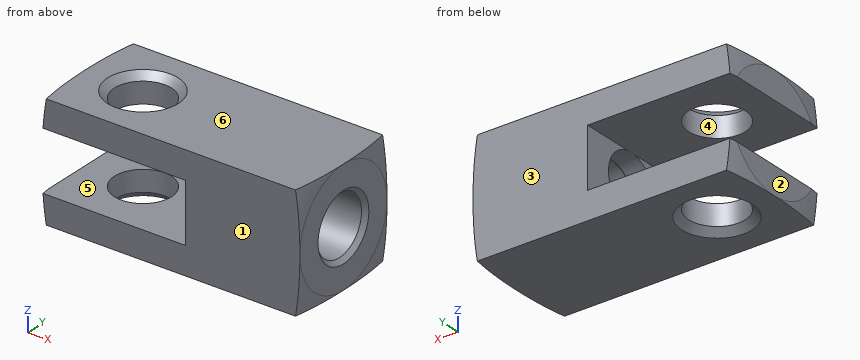
Autodesk Inventor part; units mm, degrees
ref_plane "dummy_XY" through (0, 0, 0) normal (0, 0, 1) x (1, 0, 0)
ref_plane "dummy_YZ" through (0, 0, 0) normal (1, 0, 0) x (0, 1, 0)
ref_plane "dummy_ZX" through (0, 0, 0) normal (0, 1, 0) x (0, 0, 1)
sketch "Sketch_1" plane through (0, 0, 0) normal (0, 0, 1) x (1, 0, 0)
  line L0 (-9.5504, 9.525) -> (-9.5504, -9.525)
  line L1 (-9.5504, -9.525) -> (33.3248, -9.525)
  line L2 (33.3248, -9.525) -> (33.3248, 9.525)
  line L3 (33.3248, 9.525) -> (-9.5504, 9.525)
extrude "Extrusion1" add sketch "Sketch_1" along normal mid plane 19.05
sketch "Sketch_2" plane through (0, 0, 0) normal (0, 1, 0) x (-1, 0, 0)
  line L0 (9.5504, -4.9213) -> (9.5504, 4.9213)
  line L1 (9.5504, 4.9213) -> (-14.2748, 4.9213)
  line L2 (-14.2748, 4.9213) -> (-14.2748, -4.9213)
  line L3 (-14.2748, -4.9213) -> (9.5504, -4.9213)
extrude "Extrusion2" cut sketch "Sketch_2" along normal mid plane 19.05
sketch "Sketch3" plane through (33.3248, -9.525, 9.525) normal (1, 0, 0) x (0, 0, -1)
  point P0 (9.525, 9.525)
hole "Hole1" at (33.3248, 0, 0) direction (-1, 0, 0) diameter 9.7282 depth 15.748 countersink diameter 11.1125 countersink angle 90
sketch "Sketch4" plane through (17.5768, 0, 0) normal (1, 0, 0) x (0, 0, -1)
  point P0 (0, 0)
hole "Hole2" at (17.5768, 0, 0) direction (-1, 0, 0) diameter 9.9212 depth 3.302
sketch "Sketch_5" plane through (0, 0, 0) normal (1, 0, 0) x (0, 1, 0)
  line L0 (0, -9.525) -> (0, 9.525)
  line L1 (0, 9.525) -> (5.8674, 9.525)
  line L2 (5.8674, 9.525) -> (4.7244, 8.382)
  line L3 (4.7244, 8.382) -> (4.7244, -8.382)
  line L4 (4.7244, -8.382) -> (5.8674, -9.525)
  line L5 (5.8674, -9.525) -> (0, -9.525)
  line L6 (0, -9.525) -> (0, 9.525)
revolve "Revolution1" cut sketch "Sketch_5" angle 360 about axis through (0, 0, -9.525) along (0, 0, -1)
sketch "Sketch_9" plane through (0, 0, 0) normal (0, 0, 1) x (1, 0, 0)
  line L0 (42.8498, 0) -> (33.3248, 0)
  line L1 (33.3248, 0) -> (33.3248, 9.525)
  arc A0 (33.3248, 9.525) -> (30.7848, 19.05) centre (-3.664, 4.7625) ccw
  line L2 (30.7848, 19.05) -> (42.8498, 19.05)
  line L3 (42.8498, 19.05) -> (42.8498, 0)
  line L4 (42.8498, 0) -> (33.3248, 0)
revolve "Revolution2" cut sketch "Sketch_9" angle 360 about axis through (42.8498, 0, 0) along (1, 0, 0)
sketch "Sketch_10" plane through (0, 0, 0) normal (0, 0, 1) x (1, 0, 0)
  line L0 (-9.5504, 0) -> (-19.0754, 0)
  line L1 (-19.0754, 0) -> (-19.0754, 19.05)
  line L2 (-19.0754, 19.05) -> (-7.0104, 19.05)
  arc A0 (-7.0104, 19.05) -> (-9.5504, 9.525) centre (27.4384, 4.7625) ccw
  line L3 (-9.5504, 9.525) -> (-9.5504, 0)
  line L4 (-9.5504, 0) -> (-19.0754, 0)
revolve "Revolution3" cut sketch "Sketch_10" angle 360 about axis through (-9.5504, 0, 0) along (1, 0, 0)
ref_plane "dummy_XY" through (0, 0, 0) normal (0, 0, 1) x (1, 0, 0)
ref_plane "dummy_YZ" through (0, 0, 0) normal (1, 0, 0) x (0, 1, 0)
ref_plane "dummy_ZX" through (0, 0, 0) normal (0, 1, 0) x (0, 0, 1)
ref_plane "h1_XY" through (-9.5504, 9.525, 0) normal (0, 0, 1) x (1, 0, 0)
ref_plane "h1_YZ" through (-9.5504, 9.525, 0) normal (1, 0, 0) x (0, 1, 0)
ref_plane "h1_ZX" through (-9.5504, 9.525, 0) normal (0, 1, 0) x (0, 0, 1)
ref_plane "h2_XY" through (-9.5504, -9.525, 0) normal (0, 0, 1) x (1, 0, 0)
ref_plane "h2_YZ" through (-9.5504, -9.525, 0) normal (1, 0, 0) x (0, 1, 0)
ref_plane "h2_ZX" through (-9.5504, -9.525, 0) normal (0, 1, 0) x (0, 0, 1)
ref_plane "l1_XY" through (33.3248, 9.525, 0) normal (0, 0, 1) x (1, 0, 0)
ref_plane "l1_YZ" through (33.3248, 9.525, 0) normal (1, 0, 0) x (0, 1, 0)
ref_plane "l1_ZX" through (33.3248, 9.525, 0) normal (0, 1, 0) x (0, 0, 1)
ref_plane "l11_XY" through (33.3248, 9.525, 0) normal (0, 0, 1) x (1, 0, 0)
ref_plane "l11_YZ" through (33.3248, 9.525, 0) normal (1, 0, 0) x (0, 1, 0)
ref_plane "l11_ZX" through (33.3248, 9.525, 0) normal (0, 1, 0) x (0, 0, 1)
ref_plane "l12_XY" through (0, 9.525, 0) normal (0, 0, 1) x (1, 0, 0)
ref_plane "l12_YZ" through (0, 9.525, 0) normal (1, 0, 0) x (0, 1, 0)
ref_plane "l12_ZX" through (0, 9.525, 0) normal (0, 1, 0) x (0, 0, 1)
ref_plane "l2_XY" through (-9.5504, 9.525, 0) normal (0, 0, 1) x (1, 0, 0)
ref_plane "l2_YZ" through (-9.5504, 9.525, 0) normal (1, 0, 0) x (0, 1, 0)
ref_plane "l2_ZX" through (-9.5504, 9.525, 0) normal (0, 1, 0) x (0, 0, 1)
ref_plane "l21_XY" through (33.3248, 0, 0) normal (0, 1, 0) x (1, 0, 0)
ref_plane "l21_YZ" through (33.3248, 0, 0) normal (1, 0, 0) x (0, 0, -1)
ref_plane "l21_ZX" through (33.3248, 0, 0) normal (0, 0, -1) x (0, 1, 0)
ref_plane "l22_XY" through (14.2748, 0, 0) normal (0, 1, 0) x (1, 0, 0)
ref_plane "l22_YZ" through (14.2748, 0, 0) normal (1, 0, 0) x (0, 0, -1)
ref_plane "l22_ZX" through (14.2748, 0, 0) normal (0, 0, -1) x (0, 1, 0)
ref_plane "piston_rod_clevis_XY" through (33.3248, 0, 0) normal (1, 0, 0) x (0, 0, -1)
ref_plane "piston_rod_clevis_YZ" through (33.3248, 0, 0) normal (0, 0, -1) x (0, 1, 0)
ref_plane "piston_rod_clevis_ZX" through (33.3248, 0, 0) normal (0, 1, 0) x (1, 0, 0)
ref_plane "rod_clevis_body_XY" through (0, 0, 0) normal (0, 0, 1) x (1, 0, 0)
ref_plane "rod_clevis_body_YZ" through (0, 0, 0) normal (1, 0, 0) x (0, 1, 0)
ref_plane "rod_clevis_body_ZX" through (0, 0, 0) normal (0, 1, 0) x (0, 0, 1)
ref_plane "th1_XY" through (33.3248, 5.5563, 0) normal (0, 0, 1) x (1, 0, 0)
ref_plane "th1_YZ" through (33.3248, 5.5563, 0) normal (1, 0, 0) x (0, 1, 0)
ref_plane "th1_ZX" through (33.3248, 5.5563, 0) normal (0, 1, 0) x (0, 0, 1)
ref_plane "th2_XY" through (33.3248, -5.5563, 0) normal (0, 0, 1) x (1, 0, 0)
ref_plane "th2_YZ" through (33.3248, -5.5563, 0) normal (1, 0, 0) x (0, 1, 0)
ref_plane "th2_ZX" through (33.3248, -5.5563, 0) normal (0, 1, 0) x (0, 0, 1)
ref_plane "to_cylinder_XY" through (14.2748, 0, 0) normal (1, 0, 0) x (0, 0, -1)
ref_plane "to_cylinder_YZ" through (14.2748, 0, 0) normal (0, 0, -1) x (0, 1, 0)
ref_plane "to_cylinder_ZX" through (14.2748, 0, 0) normal (0, 1, 0) x (1, 0, 0)
ref_plane "w1_XY" through (33.3248, 0, -9.525) normal (0, 1, 0) x (1, 0, 0)
ref_plane "w1_YZ" through (33.3248, 0, -9.525) normal (1, 0, 0) x (0, 0, -1)
ref_plane "w1_ZX" through (33.3248, 0, -9.525) normal (0, 0, -1) x (0, 1, 0)
ref_plane "w11_XY" through (-9.5504, 0, -4.9213) normal (0, 1, 0) x (1, 0, 0)
ref_plane "w11_YZ" through (-9.5504, 0, -4.9213) normal (1, 0, 0) x (0, 0, -1)
ref_plane "w11_ZX" through (-9.5504, 0, -4.9213) normal (0, 0, -1) x (0, 1, 0)
ref_plane "w12_XY" through (-9.5504, 0, 4.9213) normal (0, 1, 0) x (1, 0, 0)
ref_plane "w12_YZ" through (-9.5504, 0, 4.9213) normal (1, 0, 0) x (0, 0, -1)
ref_plane "w12_ZX" through (-9.5504, 0, 4.9213) normal (0, 0, -1) x (0, 1, 0)
ref_plane "w2_XY" through (33.3248, 0, 9.525) normal (0, 1, 0) x (1, 0, 0)
ref_plane "w2_YZ" through (33.3248, 0, 9.525) normal (1, 0, 0) x (0, 0, -1)
ref_plane "w2_ZX" through (33.3248, 0, 9.525) normal (0, 0, -1) x (0, 1, 0)
properties part number "D-14053" material "Steel"
Geometry: final body of the model. Coordinates: model frame, mm. Face numbers are marked on the shaded views. A direction names the side the tool comes from. Give positions to 0.01 mm unless a question says otherwise; leave off trailing zeros. Order: outer loops, then holes, each group sorted by start corner. A loop starts at its lowest first (then second) coordinate and runs counter-clockwise, first axis right, second up. Notation, with made-up numbers: (87.25, 58.25) - (139.25, 58.25) arc R14 cw to (139.25, 78.25) - close; hole circle Ø10 at (23.25, -7.5). An arc over 180 degrees is marked (long way). Use CSV: the item, a comma, the result in double quotes.
1. Mould query, pull axis Y, two halves, no side actions, for the marked faces 1, 2, 3 and 4. Classes: +Y half, -Y half, draft (parallel to the pull), parting line (faces both ways), or undercut.
Answers below:
face 1,"-Y half"
face 2,"draft"
face 3,"+Y half"
face 4,"undercut"
2. Contact query for flat-ended pins moving along their axis: pin 1 (7.5 mm diameter, centred on x = 0, y = 0, fed in from +Z); pin 2 (2.5 mm diameter, centred on y = -3.5, z = -2, fed in from -X). Output: stop coordinate, or through.
Answers below:
pin 1,"through"
pin 2,"x = 14.27"
3. Section query B-B (x = 15.5). Output: boundary loops of the cut face in (y, z) (3 decimals).
Answers below:
outline,"(-9.525, -9.525) - (9.525, -9.525) - (9.525, 9.525) - (-9.525, 9.525) - close; hole circle Ø9.921 at (0, 0)"
4. Access query for the marked faces 5 and 6. Directions: +Z, -Z, +X, -X, +Y, -Y. A direction counts if a zero-diameter tool reaches every point of the face in a straight line with its end or side. Return the directions, or none.
Answers below:
face 5,"-X, +Y, -Y"
face 6,"+Z, +X, -X, +Y, -Y"
5. Section query A-A (x = 0). Output: boundary loops of the cut face in (y, z) (3 decimals).
Answers below:
outline,"(-9.525, -9.525) - (-5.867, -9.525) - (-4.724, -8.382) - (-4.724, -4.921) - (-9.525, -4.921) - close; (-9.525, 4.921) - (-4.724, 4.921) - (-4.724, 8.382) - (-5.867, 9.525) - (-9.525, 9.525) - close; (4.724, -8.382) - (5.867, -9.525) - (9.525, -9.525) - (9.525, -4.921) - (4.724, -4.921) - close; (4.724, 4.921) - (9.525, 4.921) - (9.525, 9.525) - (5.867, 9.525) - (4.724, 8.382) - close"
6. Material intervals for line 1 along Y through (x, z) = (16.9, 0) (3 decimals); line 2 along X through (y, z) = (0, -7.3); line 3 along Z through (x, y) = (-6, -1.25) (3 decimals), sorted ascending. Write a range as from..to.
Answers below:
line 1,"-9.525..-4.961, 4.961..9.525"
line 2,"-9.55..-4.72, 4.72..33.32"
line 3,"-9.525..-4.921, 4.921..9.525"
